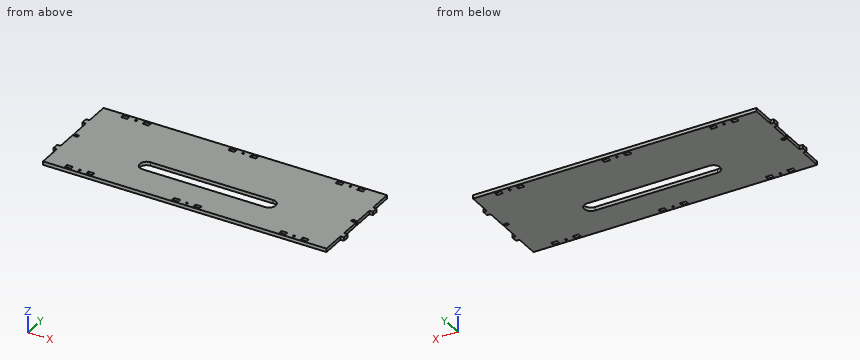
Autodesk Inventor part; units mm, degrees
ref_plane "YZ Plane" through (0, 0, 0) normal (1, 0, 0) x (0, 1, 0)
ref_plane "XZ Plane" through (0, 0, 0) normal (0, 1, 0) x (-1, 0, 0)
ref_plane "XY Plane" through (0, 0, 0) normal (0, 0, 1) x (1, 0, 0)
sketch "Sketch1" plane through (0, 0, 0) normal (0, 0, 1) x (1, 0, 0)
  line L0 (463, 164.43) -> (0, 164.43)
  line L1 (0, 164.43) -> (0, -3)
  line L2 (0, -3) -> (463, -3)
  line L3 (463, -3) -> (463, 164.43)
  point P0 (0, 0)
  point P1 (463, 161.43)
  dimension "d0" = 3
  dimension "d1" = 3
extrude "Extrusion1" add sketch "Sketch1" along normal blind 5.715
sketch "Sketch2" plane through (0, 0, 5.715) normal (0, 0, 1) x (1, 0, 0)
  line L0 (463, 164.43) -> (0, 164.43)
  line L1 (0, 164.43) -> (0, -3)
  line L2 (0, -3) -> (463, -3)
  line L3 (463, -3) -> (463, 164.43)
  line L4 (44, 0) -> (34, 0)
  line L5 (44, 5.715) -> (44, 0)
  line L6 (34, 5.715) -> (44, 5.715)
  line L7 (34, 5.715) -> (34, 0)
  line L8 (79, 0) -> (69, 0)
  line L9 (79, 5.715) -> (79, 0)
  line L10 (69, 5.715) -> (79, 5.715)
  line L11 (69, 5.715) -> (69, 0)
  line L12 (219, 0) -> (209, 0)
  line L13 (219, 5.715) -> (219, 0)
  line L14 (209, 5.715) -> (219, 5.715)
  line L15 (209, 5.715) -> (209, 0)
  line L16 (254, 0) -> (244, 0)
  line L17 (254, 5.715) -> (254, 0)
  line L18 (244, 5.715) -> (254, 5.715)
  line L19 (244, 5.715) -> (244, 0)
  line L20 (394, 0) -> (384, 0)
  line L21 (394, 5.715) -> (394, 0)
  line L22 (384, 5.715) -> (394, 5.715)
  line L23 (384, 5.715) -> (384, 0)
  line L24 (429, 0) -> (419, 0)
  line L25 (429, 5.715) -> (429, 0)
  line L26 (419, 5.715) -> (429, 5.715)
  line L27 (419, 5.715) -> (419, 0)
  line L28 (429, 155.715) -> (419, 155.715)
  line L29 (429, 161.43) -> (429, 155.715)
  line L30 (419, 161.43) -> (429, 161.43)
  line L31 (419, 161.43) -> (419, 155.715)
  line L32 (394, 155.715) -> (384, 155.715)
  line L33 (394, 161.43) -> (394, 155.715)
  line L34 (384, 161.43) -> (394, 161.43)
  line L35 (384, 161.43) -> (384, 155.715)
  line L36 (254, 155.715) -> (244, 155.715)
  line L37 (254, 161.43) -> (254, 155.715)
  line L38 (244, 161.43) -> (254, 161.43)
  line L39 (244, 161.43) -> (244, 155.715)
  line L40 (219, 155.715) -> (209, 155.715)
  line L41 (219, 161.43) -> (219, 155.715)
  line L42 (209, 161.43) -> (219, 161.43)
  line L43 (209, 161.43) -> (209, 155.715)
  line L44 (79, 155.715) -> (69, 155.715)
  line L45 (79, 161.43) -> (79, 155.715)
  line L46 (69, 161.43) -> (79, 161.43)
  line L47 (69, 161.43) -> (69, 155.715)
  line L48 (44, 155.715) -> (34, 155.715)
  line L49 (44, 161.43) -> (44, 155.715)
  line L50 (34, 161.43) -> (44, 161.43)
  line L51 (34, 161.43) -> (34, 155.715)
  point P0 (0, 0)
extrude "Extrusion2" cut sketch "Sketch2" against normal through all keep common part
sketch "Sketch3" plane through (0, 0, 5.715) normal (0, 0, 1) x (1, 0, 0)
  line L0 (44, 155.715) -> (44, 161.43)
  line L1 (69, 161.43) -> (69, 155.715)
  line L2 (219, 155.715) -> (219, 161.43)
  line L3 (244, 161.43) -> (244, 155.715)
  line L4 (394, 155.715) -> (394, 161.43)
  line L5 (419, 161.43) -> (419, 155.715)
  line L6 (419, 5.715) -> (419, 0)
  line L7 (394, 0) -> (394, 5.715)
  line L8 (244, 5.715) -> (244, 0)
  line L9 (219, 0) -> (219, 5.715)
  line L10 (69, 5.715) -> (69, 0)
  line L11 (44, 0) -> (44, 5.715)
  line L12 (44, 158.5725) -> (69, 158.5725) construction
  circle A0 centre (56.5, 158.5725) radius 1.5
  line L13 (219, 158.5725) -> (244, 158.5725) construction
  circle A1 centre (231.5, 158.5725) radius 1.5
  line L14 (394, 158.5725) -> (419, 158.5725) construction
  circle A2 centre (406.5, 158.5725) radius 1.5
  line L15 (44, 2.8575) -> (69, 2.8575) construction
  circle A3 centre (56.5, 2.8575) radius 1.5
  line L16 (219, 2.8575) -> (244, 2.8575) construction
  circle A4 centre (231.5, 2.8575) radius 1.5
  line L17 (394, 2.8575) -> (419, 2.8575) construction
  circle A5 centre (406.5, 2.8575) radius 1.5
  point P0 (0, 0)
  dimension "d6" = 3
  dimension "d8" = 3
  dimension "d9" = 3
  dimension "d10" = 3
  dimension "d11" = 3
  dimension "d12" = 3
extrude "Extrusion3" cut sketch "Sketch3" against normal through all
sketch "Sketch4" plane through (0, 0, 5.715) normal (0, 0, 1) x (1, 0, 0)
  line L0 (0, 164.43) -> (0, -3)
  line L1 (0, 82.215) -> (8.285, 82.215)
  line L2 (8.285, 82.215) -> (8.285, 79.215)
  line L3 (8.285, 79.215) -> (0, 79.215)
  line L4 (0, 79.215) -> (0, 82.215)
  line L5 (4.285, 83.465) -> (6.285, 83.465)
  line L6 (6.285, 83.465) -> (6.285, 77.965)
  line L7 (6.285, 77.965) -> (4.285, 77.965)
  line L8 (4.285, 77.965) -> (4.285, 83.465)
  point P0 (0, 0)
  point P1 (0, 80.715)
  point P2 (6.285, 80.715)
  point P3 (8.285, 80.715)
  dimension "d15" = 3
  dimension "d17" = 5.5
  dimension "d18" = 6.285
  dimension "d19" = 2
  dimension "d20" = 8.285
extrude "Extrusion4" cut sketch "Sketch4" against normal through all
ref_plane "Work Plane1" through (231.5, 164.43, 0) normal (-1, 0, 0) x (0, 0, 1)
sketch "Sketch5" plane through (0, 0, 5.715) normal (0, 0, 1) x (1, 0, 0)
  line L0 (0, 79.215) -> (0, -3)
  line L1 (0, 164.43) -> (0, 82.215)
  line L2 (8.285, 82.215) -> (8.285, 79.215)
  line L3 (0, 125.715) -> (-5.715, 125.715)
  line L4 (-5.715, 125.715) -> (-5.715, 115.715)
  line L5 (-5.715, 115.715) -> (0, 115.715)
  line L6 (0, 115.715) -> (0, 125.715)
  line L7 (0, 45.715) -> (-5.715, 45.715)
  line L8 (-5.715, 45.715) -> (-5.715, 35.715)
  line L9 (-5.715, 35.715) -> (0, 35.715)
  line L10 (0, 35.715) -> (0, 45.715)
  line L11 (-5.715, 45.715) -> (-5.715, 115.715)
  point P0 (0, 0)
  point P1 (8.285, 80.715)
  point P2 (-5.715, 80.715)
  point P3 (8.285, 80.715)
  dimension "d23" = 35
  dimension "d26" = 5.715
  dimension "d27" = 10
extrude "Extrusion5" add sketch "Sketch5" against normal up to surface (5.715 mm away)
mirror "Mirror1" about plane through (231.5, 164.43, 0) normal (-1, 0, 0) of "Extrusion5", "Extrusion4"
sketch "Sketch6" plane through (0, 0, 5.715) normal (0, 0, 1) x (1, 0, 0)
  circle A0 centre (231.5, 2.8575) radius 1.5
  line L0 (356, 95.715) -> (341, 95.715)
  line L1 (341, 25.715) -> (356, 25.715)
  line L2 (348.5, 25.715) -> (348.5, 95.715)
  line L3 (331.5, 49.715) -> (131.5, 49.715)
  arc A1 (131.5, 71.715) -> (131.5, 49.715) centre (131.5, 60.715) ccw
  line L4 (131.5, 71.715) -> (331.5, 71.715)
  arc A2 (331.5, 49.715) -> (331.5, 71.715) centre (331.5, 60.715) ccw
  point P0 (0, 0)
  point P1 (231.5, 49.715)
  point P2 (348.5, 60.715)
  dimension "d30" = 200
  dimension "d32" = 22
extrude "Extrusion6" cut sketch "Sketch6" against normal through all contours L3 A1 L4 A2
properties part number "TOP PLATE"
Part model, mm, in its own coordinate system. Round coordinates to 2 decimals unless told otherwise and drop trailing zeros. Loops run counter-clockwise (first coordinate to the right, second up) from the corner with the lowest first, then second, coordinate; pieces in that order, holes last.
1. Slice it at A-A (x = 277). Give the cut face in (y, z) (3 decimals).
Solutions:
outline: (-3, 0) - (49.715, 0) - (49.715, 5.715) - (-3, 5.715) - close; (71.715, 0) - (164.43, 0) - (164.43, 5.715) - (71.715, 5.715) - close
2. Flat gauge pins, fed straight in: pin 1 (1.7 mm diameter, centred on y = 4, z = 3, fed in from -X); pin 2 (1.4 mm diameter, centred on y = 78.5, z = 2.5, fed in from +X); pin 3 (2.5 mm diameter, centred on x = 56.5, y = 2.86, fed in from +Z); pin 4 (1.7 mm diameter, centred on x = -1.5, z = 4, fed in from -Y) (3 decimals). Where does each tip first touch, or does it go through?
Solutions:
pin 1: stops at x = 0
pin 2: stops at x = 463
pin 3: passes through
pin 4: stops at y = 35.715
3. Slice it at C-C (z = 2.7). Count the separate pieces of the cut face and the enclosed holes in it, and give its area (3 significant figures).
Solutions:
separate pieces: 1
enclosed holes: 19
area: 72,200 mm2
4. Slice it at B-B (y = 93). Give the cut face in (x, z) (3 decimals).
Solutions:
outline: (0, 0) - (463, 0) - (463, 5.715) - (0, 5.715) - close
5. Drill centre lines: line 1 along Y through (x, z) = (386.5, 4.4) (3 decimals); line 2 along Y through (x, z) = (56.5, 3.6); line 3 along Y through (x, z) = (231.5, 2.45) (1 decimal). Where is each one in solid material? Low to high.
Solutions:
line 1: y = -3 to 0, 5.715 to 155.715, 161.43 to 164.43
line 2: y = -3 to 1.36, 4.36 to 157.07, 160.07 to 164.43
line 3: y = -3 to 1.4, 4.4 to 49.7, 71.7 to 157.1, 160.1 to 164.4
